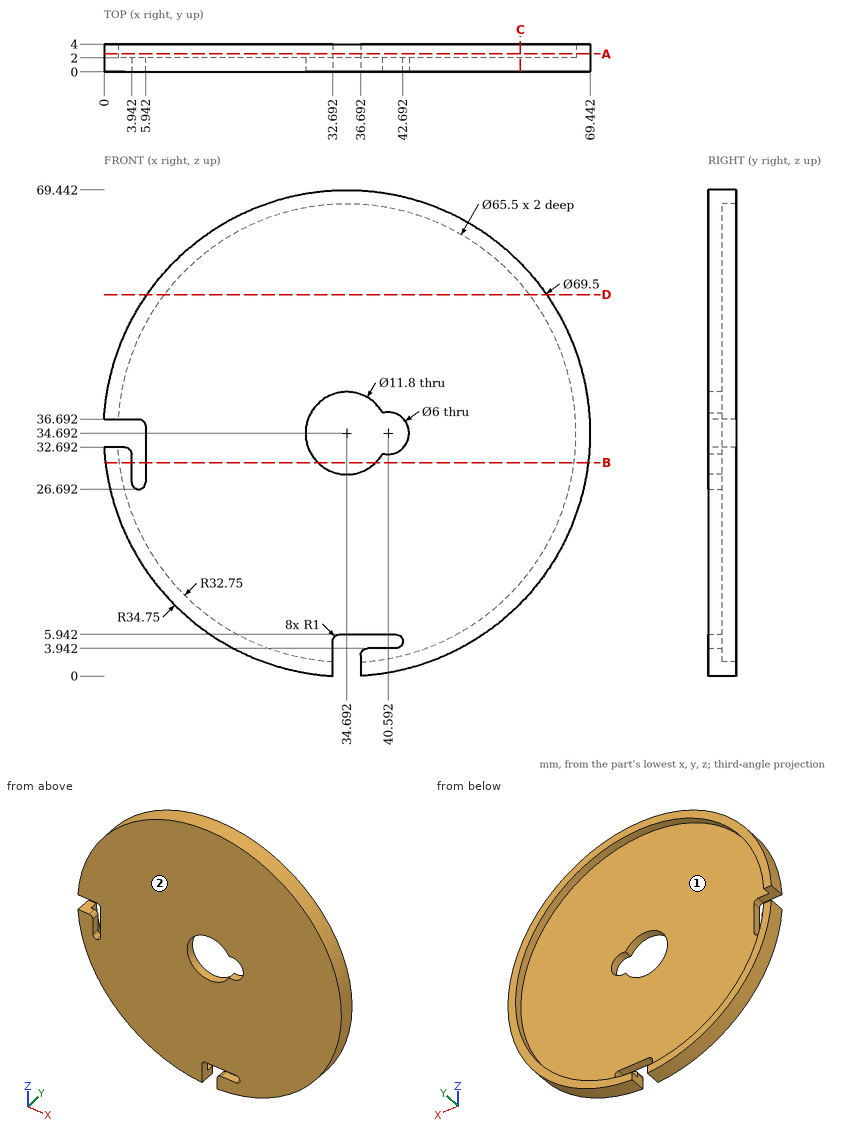
Answer from the drawing. Dimensions are ordinates in mm from the lowest x, y and z of the part. Give positions to 0.01 mm unless a question says otherwise; leave off trailing zeros. Loops run counter-clockwise (first coordinate to the right, second up) from the corner with the lowest first, then second, coordinate; pieces in that order, holes last. Notation, with made-up numbers: (47, 81.25) - (75, 81.25) arc R5 ccw to (75, 89.25) - close; hole circle Ø6 at (64.25, -37). An arc over 180 degrees is marked (long way). Answer as a JSON object with one key per item and string values.
1. A cutting plane is placed at B-B (z = 30.5). Write down the section's boundary in (x, y).
Determined:
{"outline": "(0.2, 0) - (3.94, 0) - (3.94, 2) - (2.21, 2) - (2.21, 4) - (0.2, 4) - close; (5.94, 0) - (30.54, 0) - (30.54, 2) - (5.94, 2) - close; (38.84, 0) - (69.19, 0) - (69.19, 4) - (67.17, 4) - (67.17, 2) - (38.84, 2) - close"}
2. A cutting plane is placed at C-C (x = 59.5). Write down the section's boundary in (y, z).
Determined:
{"outline": "(0, 10.36) - (4, 10.36) - (4, 13.31) - (2, 13.31) - (2, 56.07) - (4, 56.07) - (4, 59.03) - (0, 59.03) - close"}
3. Flat-ended cylindrical pins translate along their axes: pin 1 Ø2 at (y, z) = (0.5, 31.5) entering from -X; pin 2 Ø12 at (x, z) = (34, 36.5) entering from +Y; pin 3 Ø5 at (x, z) = (27.5, 31.5) entering from -Y; pin 4 Ø1.6 at (x, y) = (39, 1) entering from +Z (1 decimal). Find the tip coordinate at first contact, or state that the pin passes through.
Determined:
{"pin 1": "x = 0.01", "pin 2": "y = 2", "pin 3": "y = 0", "pin 4": "z = 69.3"}
4. A cutting plane is placed at A-A (y = 2.6). Write down the section's boundary in (x, z), then the cut area to 3 significant figures.
Determined:
{"outline": "(0, 32.69) arc R34.75 ccw to (32.69, 0) - (32.69, 2) arc R32.75 cw to (2, 32.69) - close; (0, 36.69) - (2, 36.69) arc R32.75 cw (long way) to (36.69, 2) - (36.69, 0) arc R34.75 ccw (long way) to start", "area": "408 mm²"}
5. Find the intervals of material crossed by L1, parallel to Y at x = 39.5, z = 28.5; L2, parallel to Z at x = 22, y = 2.6; L3, parallel to X at y = 2.75, z = 49 (1 decimal), in increasing order. Write a range as [from, to].
Determined:
{"L1": "[0, 2]", "L2": "[2.34, 4.5], [64.88, 67.04]", "L3": "[3, 5.2], [64.2, 66.4]"}
6. A cutting plane is placed at D-D (z = 54.5). Write down the section's boundary in (x, y) (1 decimal), then the cut area to 3 significant figures.
Determined:
{"outline": "(6.1, 0) - (63.2, 0) - (63.2, 4) - (60.8, 4) - (60.8, 2) - (8.6, 2) - (8.6, 4) - (6.1, 4) - close", "area": "124 mm²"}
7. For a pull along X with two mould halves and no side action, classify the marked faces 1 and 2 as pulls with the +X half, pulls with the -X half, needs draft (parallel to the pull), parting line crosses it, or undercut.
Determined:
{"face 1": "undercut", "face 2": "needs draft"}
